from build123d import *

# Parameters (mm, degrees)
F0_W     = 33
F0_H     = 33
F1_DEPTH = 500
F2_R     = 3
F3_R     = 4
F4_DEPTH = 25


with BuildPart() as f1:
    # F0 (on Top) → F1 (new body)
    with BuildSketch(Plane.XY):
        with Locations((16.5, -16.5)):
            Rectangle(F0_W, F0_H)
    extrude(amount=F1_DEPTH)

    # F2
    f2_edges = [f1.edges().sort_by_distance(p)[0] for p in [
        (33, 0, 250),
        (33, -33, 250),
        (0, -33, 250),
        (0, 0, 250),
    ]]
    fillet(f2_edges, radius=F2_R)

    # F3 (on face) → F4 (cut)
    with BuildSketch(Plane(origin=(0, 0, 0), x_dir=(1, 0, 0), z_dir=(0, 0, -1))):
        with Locations((16.5, 16.5)):
            Circle(F3_R)
    extrude(amount=-F4_DEPTH, mode=Mode.SUBTRACT)


solid = f1.part
Check sheet for the modelled part. Datum: model origin and axes. Units: mm. A direction names the side the tool comes from. Round coordinates to 2 decimals unless told otherwise and drop trailing zeros. Put each result on its own line as item: value. Start each with the question number.
1. Gauge pin test, flat end, axial feed: pin 1 (2 mm diameter, centred on x = 15.5, y = -17.5, fed in from -Z). Record the tip position at first contact, or that the pin passes through.
2. Scan lines: probe 1 along X at (y, z) = (-16.5, 8.25); probe 2 along Y at (x, z) = (16, 11); probe 3 along Z at (x, y) = (17, -15.5). Record each from-to range of solid material in increasing order.
3. Access from +Z, -Z, +X, -X, +Y, -Y to the whole of each face (thin tool, end or side, straight path). Record for faces 1 (the face through (16, -17, 25)), 2 (the face through (16, 0, 246)).
4. Draft check along X on faces 3 (the face through (33, -17, 246)), 4 (the face through (13.55, -19.2, 12.32)), 5 (the face through (16, -16, 500)). Enter one of: +X half, -X half, draft (parallel to the pull), parting line (faces both ways), or undercut.
Findings:
1. pin 1: stops at z = 25
2. probe 1: x = 0 to 12.5, 20.5 to 33
2. probe 2: y = -33 to -20.47, -12.53 to 0
2. probe 3: z = 25 to 500
3. face 1: -Z
3. face 2: +Z, -Z, +X, -X, +Y
4. face 3: +X half
4. face 4: undercut
4. face 5: draft
